Read the model definition and answer for the solid it produces. Units are mm, in the model's axes. A direction names the side the tool comes from. Round coordinates to 2 decimals unless told otherwise and drop trailing zeros. Order: outer loops, then holes, each group sorted by start corner. A loop starts at its lowest first (then second) coordinate and runs counter-clockwise, first axis right, second up. Notation, with made-up numbers: (42.25, 83.5) - (93.25, 83.5) arc R12 ccw to (93.25, 106.5) - close; hole circle Ø8 at (-2, -3). An arc over 180 degrees is marked (long way). Answer as a JSON object with one key per item and string values. Group by question number.
Q1. A cutting plane is placed at A-A on z = -13.75. Determine the outline of the cut face in (x, y).
Q2. A tool of negligible diameter and unlimited length cuts with its end or side. For faces 4 (the flat face through (2, 0, 0)), 5 (the flat face through (-2.8, -2.7, -11.8)), 6 (the flat face through (9.8, 1.5, -3.5)), 7 (the flat face through (-5.208, 1.528, -1.43)), 8 (the flat face through (9.8, -1.5, -3.5)), from which of +Z, -Z, +X, -X, +Y, -Y can it reach the whole face along a straight path? Write none if from no direction.
Q3. Consider line 1 (Y direction, x = 5.5, z = 0); line 2 (Y direction, x = 4, z = -13.25); line 3 (Z direction, x = -6.75, y = 0). Determine where each line is inside the solid, lowest interval first.
Q4. A cutting plane is placed at C-C on x = 7.5. Determine the outline of the cut face in (y, z).
Q5. Given pin 1 Ø1 at (y, z) = (-0.5, 0.5) entering from +X; pin 2 Ø4 at (x, z) = (12.5, -12) entering from -Y; pin 3 Ø1 at (y, z) = (-2, -8.5) entering from +X; pin 4 Ø2 at (y, z) = (0, -11) entering from -X, each flat-ended and moving along its own axis, determine where each tip first touches the part or whether it passes through.
Q6. A cutting plane is placed at D-D on z = 0. Determine the outline of the cut face in (x, y).
Q7. A cutting plane is placed at B-B on y = -2.5. Determine the outline of the cut face in (x, z).
Q8. The mould has two halves that part along X. Classify faces 1 (the flat face through (2.8, -2.7, -8.9)), 2 (the flat face through (-3.5, 0, -12)), 3 (the flat face through (-7, 2, -6.5)): pulls with the +X half, pulls with the -X half, needs draft (parallel to the pull), parting line crosses it, or undercut.
```python
from build123d import *

# Parameters (mm, degrees)
BOSS_EXTRUDE1_DEPTH  = 3.5
SKETCH2_R            = 1.6
CUT_EXTRUDE1_DEPTH   = 14
SKETCH3_R            = 1.6
CUT_EXTRUDE2_DEPTH   = 14
BOSS_EXTRUDE2_DEPTH  = 1
BOSS_EXTRUDE13_START = -19.5
BOSS_EXTRUDE13_DEPTH = 10
BOSS_EXTRUDE14_DEPTH = 1
CHAMFER7_SIZE        = 1.5


with BuildPart() as part:
    # Sketch1 → Boss-Extrude1 (new, symmetric)
    with BuildSketch(Plane(origin=(0, 0, 0), x_dir=(1, 0, 0), z_dir=(0, 1, 0))):
        Polygon((-3.5, 16), (-3.5, -3.5), (16, -3.5), (16, 3.5), (3.5, 3.5), (3.5, 16), align=None)
    extrude(amount=BOSS_EXTRUDE1_DEPTH, both=True)

    # Sketch2 → Cut-Extrude1 (cut)
    with BuildSketch(Plane(origin=(0, 0, -16), x_dir=(-1, 0, 0), z_dir=(0, 0, -1))):
        Circle(SKETCH2_R)
    extrude(amount=-CUT_EXTRUDE1_DEPTH, mode=Mode.SUBTRACT)

    # Sketch3 → Cut-Extrude2 (cut)
    with BuildSketch(Plane(origin=(16, 0, 0), x_dir=(0, 0, -1), z_dir=(1, 0, 0))):
        Circle(SKETCH3_R)
    extrude(amount=-CUT_EXTRUDE2_DEPTH, mode=Mode.SUBTRACT)

    # Sketch4 → Boss-Extrude2 (add, symmetric)
    with BuildSketch(Plane(origin=(0, 0, 0), x_dir=(1, 0, 0), z_dir=(0, 1, 0))):
        Polygon((3.5, 16), (16, 3.5), (3.5, 3.5), align=None)
    extrude(amount=BOSS_EXTRUDE2_DEPTH, both=True)

    # Sketch16 → Boss-Extrude13 (add)
    with BuildSketch(Plane(origin=(0, 0, -16), x_dir=(-1, 0, 0), z_dir=(0, 0, -1)).offset(BOSS_EXTRUDE13_START)):
        Polygon((3.5, -3.5), (3.5, 3.5), (5.555307923, 3.5), (4.85, -0.5), (9.15, -0.5), (8.444692077, 3.5), (10.5, 3.5), (10.5, -3.5), align=None)
    extrude(amount=BOSS_EXTRUDE13_DEPTH)

    # Sketch17 → Boss-Extrude14 (add)
    with BuildSketch(Plane(origin=(0, 0, -6.5), x_dir=(-1, 0, 0), z_dir=(0, 0, -1))):
        Polygon((5.555307923, 3.5), (3.5, 3.5), (3.5, -3.5), (10.5, -3.5), (10.5, 3.5), (8.444692077, 3.5), (9.15, -0.5), (4.85, -0.5), align=None)
        Polygon((9.15, -0.5), (8.444692077, 3.5), (5.555307923, 3.5), (4.85, -0.5), align=None)
    extrude(amount=BOSS_EXTRUDE14_DEPTH)

    # Chamfer7
    chamfer7_edges = [part.edges().sort_by_distance(p)[0] for p in [
        (5.222346039, 3.5, 3.5),
        (9.75, 3.5, -3.5),
        (3.5, 3.5, -9.75),
        (-10.5, -3.5, -2),
        (-9.472346039, 3.5, 3.5),
        (0, 3.5, -16),
        (3.5, -3.5, -9.75),
        (9.75, -3.5, -3.5),
        (2.75, -3.5, 3.5),
        (-3.5, -3.5, -11.75),
        (-3.5, 3.5, -11.75),
    ]]
    chamfer(chamfer7_edges, length=CHAMFER7_SIZE)


solid = part.part
```
Result set:
{
 "1": {"outline": "(-3.5, -2) - (-2, -3.5) - (2, -3.5) - (3.5, -2) - (3.5, -1) - (5.75, -1) - (5.75, 1) - (3.5, 1) - (3.5, 2) - (2, 3.5) - (-2, 3.5) - (-3.5, 2) - close; hole circle Ø3.2 at (0, 0)"},
 "2": {"face 4": "+X", "face 5": "-Z, -X, -Y", "face 6": "-Z, +X, +Y", "face 7": "+Z", "face 8": "-Z, +X, -Y"},
 "3": {"line 1": "y = -3.5 to -1.6, 1.6 to 3.5", "line 2": "y = -1 to 1", "line 3": "z = -7.5 to -6.5"},
 "4": {"outline": "(-3.5, -2) - (-2, -3.5) - (-1, -3.5) - (-1, -12) - (1, -12) - (1, -3.5) - (2, -3.5) - (3.5, -2) - (3.5, 2) - (2, 3.5) - (-2, 3.5) - (-3.5, 2) - close; hole circle Ø3.2 at (0, 0)"},
 "5": {"pin 1": "stops at x = 2", "pin 2": "passes through", "pin 3": "stops at x = 3.5", "pin 4": "stops at x = -3.5"},
 "6": {"outline": "(-10.5, -2) - (-9, -3.5) - (16, -3.5) - (16, -1.6) - (2, -1.6) - (2, 1.6) - (16, 1.6) - (16, 3.5) - (-5.56, 3.5) - (-4.85, -0.5) - (-9.15, -0.5) - (-8.44, 3.5) - (-10.5, 3.5) - close"},
 "7": {"outline": "(-10, -7.5) - (-3, -7.5) - (-3, -16) - (3, -16) - (3, -3) - (16, -3) - (16, 3) - (-10, 3) - close"},
 "8": {"face 1": "pulls with the +X half", "face 2": "pulls with the -X half", "face 3": "undercut"}
}
